Input: part model. Units: mm. Frame: model coordinates. A direction names the side the tool comes from. Coordinates: 2 decimals unless noted, no trailing zeros. Write each loop counter-clockwise with the first axis right and the second up, starting at its lowest first coordinate (ties: lowest second). Pieces come first, ordered by that corner, then holes. Notation, with made-up numbers: (56.25, 67) - (73.25, 67) arc R18 ccw to (73.25, 95) - close; hole circle Ø7 at (75, 51). An arc over 180 degrees is marked (long way). Put each result on its own line as item: value. Start each with the question number.
1. Cut plane D-D, the plane x = -14. Return loops of the section in (y, z), and give its area (3 significant figures).
2. Cut plane C-C, the plane x = 30.3. Return loops of the section in (y, z), and give its area (3 significant figures).
3. Cut plane A-A, the plane y = 1. Return loops of the section in (x, z), and give its area (3 significant figures).
4. Access query for faces 1 (the cylindrical face through (-43.751, 0.336, -67.286)), 2 (the cylindrical face through (43.751, 0.336, 67.286)). Directions: +Z, -Z, +X, -X, +Y, -Y. A direction counts if a zero-diameter tool reaches every point of the face in a straight line with its end or side. Return the directions, or none.
5. Pull-direction query (X, two-part tool) for faces 3 (the cylindrical face through (-30.099, 0.336, 69.798)), 4 (the cylindrical face through (44.11, 0.34, 67.22)); classes: released by +X, released by -X, zero draft, split by the parting line, or undercut.
6. Cut plane B-B, the plane z = 59. Return loops of the section in (x, y).
7. Pin query (flat end, axial travel): pin 1 (6 mm diameter, centred on x = -27, y = 9.5, fed in from +Z); pin 2 (3 mm diameter, centred on y = 7, z = 5.5, fed in from -X); pin 3 (1.5 mm diameter, centred on x = -14.5, y = 7, fed in from +Z). Return the tip coordinate at first contact, or that it passes through.
8. Line query: line 1 (X direction, y = -18, z = 45.5); line 2 (X direction, y = 6.5, z = 32); line 3 (Z direction, x = 31.5, y = -18). Output: solid intervals per line, ascending.
from build123d import *

# Parameters (mm, degrees)
BOSS_EXTRUDE1_DEPTH = 24


with BuildPart() as part:
    # Sketch1 → Boss-Extrude1 (new, symmetric)
    with BuildSketch(Plane(origin=(0, 0, 0), x_dir=(1, 0, 0), z_dir=(0, 1, 0))):
        with BuildLine():
            Line((-41.300703165, 60.713744192), (-39.799273906, -60.717453242))
            ThreePointArc((-39.799273906, -60.717453242), (-30.3, -70.1), (-20.800726094, -60.717453242))
            Line((-20.800726094, -60.717453242), (-19.299296835, 60.713744192))
            ThreePointArc((-19.299296835, 60.713744192), (-10.1, 69.8), (-0.900703165, 60.713744192))
            Line((-0.900703165, 60.713744192), (0.600726094, -60.717453242))
            ThreePointArc((0.600726094, -60.717453242), (10.1, -70.1), (19.599273906, -60.717453242))
            Line((19.599273906, -60.717453242), (21.100703165, 60.713744192))
            ThreePointArc((21.100703165, 60.713744192), (30.3, 69.8), (39.499296835, 60.713744192))
            Line((39.499296835, 60.713744192), (41.000726094, -60.717453242))
            ThreePointArc((41.000726094, -60.717453242), (43.824140722, -67.358912849), (50.5, -70.1))
            Line((50.5, -70.1), (50.5, -69.8))
            ThreePointArc((50.5, -69.8), (44.034957331, -67.145473496), (41.300703165, -60.713744192))
            Line((41.300703165, -60.713744192), (39.799273906, 60.717453242))
            ThreePointArc((39.799273906, 60.717453242), (30.3, 70.1), (20.800726094, 60.717453242))
            Line((20.800726094, 60.717453242), (19.299296835, -60.713744192))
            ThreePointArc((19.299296835, -60.713744192), (10.1, -69.8), (0.900703165, -60.713744192))
            Line((0.900703165, -60.713744192), (-0.600726094, 60.717453242))
            ThreePointArc((-0.600726094, 60.717453242), (-10.1, 70.1), (-19.599273906, 60.717453242))
            Line((-19.599273906, 60.717453242), (-21.100703165, -60.713744192))
            ThreePointArc((-21.100703165, -60.713744192), (-30.3, -69.8), (-39.499296835, -60.713744192))
            Line((-39.499296835, -60.713744192), (-41.000726094, 60.717453242))
            ThreePointArc((-41.000726094, 60.717453242), (-43.824140722, 67.358912849), (-50.5, 70.1))
            Line((-50.5, 70.1), (-50.5, 69.8))
            ThreePointArc((-50.5, 69.8), (-44.034957331, 67.145473496), (-41.300703165, 60.713744192))
        make_face()
    extrude(amount=BOSS_EXTRUDE1_DEPTH, both=True)


solid = part.part
Report:
1. outline: (-24, -69.26) - (24, -69.26) - (24, -68.93) - (-24, -68.93) - close
1. area: 15.8 mm^2
2. outline: (-24, -70.1) - (24, -70.1) - (24, -69.8) - (-24, -69.8) - close
2. area: 14.4 mm^2
3. outline: (-50.5, -70.1) arc R9.5 ccw to (-41, -60.72) - (-39.5, 60.71) arc R9.2 cw to (-21.1, 60.71) - (-19.6, -60.72) arc R9.5 ccw to (-0.6, -60.72) - (0.9, 60.71) arc R9.2 cw to (19.3, 60.71) - (20.8, -60.72) arc R9.5 ccw to (39.8, -60.72) - (41.3, 60.71) arc R9.2 cw to (50.5, 69.8) - (50.5, 70.1) arc R9.5 ccw to (41, 60.72) - (39.5, -60.71) arc R9.2 cw to (21.1, -60.71) - (19.6, 60.72) arc R9.5 ccw to (0.6, 60.72) - (-0.9, -60.71) arc R9.2 cw to (-19.3, -60.71) - (-20.8, 60.72) arc R9.5 ccw to (-39.8, 60.72) - (-41.3, -60.71) arc R9.2 cw to (-50.5, -69.8) - close
3. area: 226 mm^2
4. face 1: -Z, +Y, -Y
4. face 2: +Z, +Y, -Y
5. face 3: undercut
5. face 4: released by +X
6. outline: (-39.82, -24) - (-39.52, -24) - (-39.52, 24) - (-39.82, 24) - close; (-21.08, -24) - (-20.78, -24) - (-20.78, 24) - (-21.08, 24) - close; (0.58, -24) - (0.88, -24) - (0.88, 24) - (0.58, 24) - close; (19.32, -24) - (19.62, -24) - (19.62, 24) - (19.32, 24) - close; (40.98, -24) - (41.28, -24) - (41.28, 24) - (40.98, 24) - close
7. pin 1: stops at z = 70.1
7. pin 2: stops at x = -40.5
7. pin 3: stops at z = -68.22
8. line 1: x = -39.99 to -39.69, -20.91 to -20.61, 0.41 to 0.71, 19.49 to 19.79, 40.81 to 41.11
8. line 2: x = -40.15 to -39.85, -20.75 to -20.45, 0.25 to 0.55, 19.65 to 19.95, 40.65 to 40.95
8. line 3: z = -70.02 to -69.72
